Autodesk Fusion 360 part; units mm, degrees
sketch "Baza" plane through (0, 0, 0) normal (0, 0, 1) x (1, 0, 0)
  line L0 (33, 21) -> (-33, 21)
  line L1 (-33, 21) -> (-33, -21)
  line L2 (-33, -21) -> (33, -21)
  line L3 (33, -21) -> (33, 21)
  line L4 (33, 21) -> (-33, -21) construction
  line L5 (-33, 21) -> (33, -21) construction
  dimension "d1" = 42
  dimension "d2" = 66
extrude "Extrude1" add sketch "Baza" along normal blind 12
chamfer "Chamfer1" distance 12 angle 45 2 edges at (33, -21, 6) (33, 21, 6)
sketch "Baza 2" plane through (0, 0, 12) normal (0, 0, 1) x (-1, 0, 0)
  line L0 (-33, -9) -> (-21, -21)
  line L1 (-21, -21) -> (33, -21)
  line L2 (33, -21) -> (33, 21)
  line L3 (33, 21) -> (-21, 21)
  line L4 (-21, 21) -> (-33, 9)
  line L5 (-33, 9) -> (-33, -9)
  line L6 (33, -21) -> (21, -21)
  line L7 (21, -21) -> (21, 21)
  line L8 (21, 21) -> (33, 21)
  line L9 (33, 21) -> (33, -21)
  dimension "d9" = 12
extrude "Extrude3" add sketch "Baza 2" along normal blind 48 contours L1 L2 L3 L6 L7 L8 L9
fillet "Fillet1" radius 21 2 edges at (-27, -21, 60) (-27, 21, 60)
sketch "Triunghi" plane through (0, 0, 0) normal (0, 1, 0) x (1, 0, 0)
  line L0 (-20.989, -53.9545) -> (-20.989, -11.9545)
  line L1 (-20.989, -11.9545) -> (33.011, -11.9545)
  line L2 (33.011, -11.9545) -> (-20.989, -53.9545)
  dimension "d14" = 42
  dimension "d15" = 54
extrude "Extrude4" add sketch "Triunghi" along normal mid plane 12
equation "d10 = 60 mm - 12 mm"
equation "d15 = 66 mm - 12 mm"
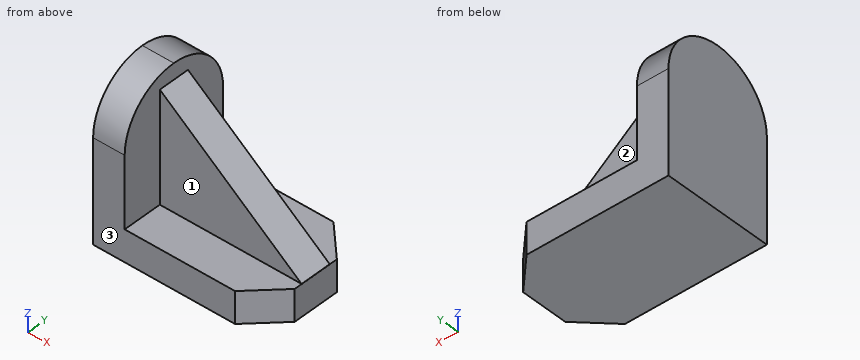
Source: CAD feature listing. Evaluate the final solid. Frame: model axes, mm. Face numbers are marked on the shaded views. A direction names the side the tool comes from. Round coordinates to 2 decimals unless told otherwise and drop trailing zeros. Loops run counter-clockwise (first coordinate to the right, second up) from the corner with the lowest first, then second, coordinate; pieces in that order, holes last. Notation, with made-up numbers: M 34,78 L 42,78 A25 ccw 42,94 Z; hole C 17,60.25 d6. An arc over 180 degrees is marked long. Use a Markdown table: item, result. Add a question column.
1. Set-up query: the marked faces 1, 2 and 3. Return all of +Z, -Z, +X, -X, +Y, -Y with unobstructed straight access to the full face (end or side cutting, diameter ignored); none if empty.
2. Ray query, line 1 along Z through (x, y) = (26.5, 7); line 2 along Y through (x, z) = (-2, 34); line 3 along X through (y, z) = (-15, 50). Return the intervals inside material, ascending. Write a range as [from, to].
3. Cut plane A-A, the plane z = 29. Output: boundary loops of the cut face in (x, y), and give its area (3 significant figures).
4. Cut plane D-D, the plane z = 13.5. Output: boundary loops of the cut face in (x, y).
5. Contact query for flat-ended pins moving along their axis: pin 1 (1.5 mm diameter, centred on x = 23.5, z = 8, fed in from +Y); pin 2 (9.5 mm diameter, centred on y = 4, z = 7, fed in from +X); pin 3 (21 mm diameter, centred on y = -2.5, z = 36.5, fed in from +X). Output: stop coordinate, or through.
Solution:
| question | item | result |
|---|---|---|
| 1 | face 1 | +Z, +X, -Y |
| 1 | face 2 | +Z, +X, +Y |
| 1 | face 3 | +Z, -Z, +X, -X, -Y |
| 2 | line 1 | z = [0, 12] |
| 2 | line 2 | y = [-6, 6] |
| 2 | line 3 | x = [-33, -21] |
| 3 | outline | M -33,-21 L -21,-21 L -21,21 L -33,21 Z; M -20.99,-6 L 11.1,-6 L 11.1,6 L -20.99,6 Z |
| 3 | area | 889 mm2 |
| 4 | outline | M -33,-21 L -21,-21 L -21,21 L -33,21 Z; M -20.99,-6 L 31.02,-6 L 31.02,6 L -20.99,6 Z |
| 5 | pin 1 | stops at y = 19.25 |
| 5 | pin 2 | stops at x = 33 |
| 5 | pin 3 | stops at x = 14.95 |
